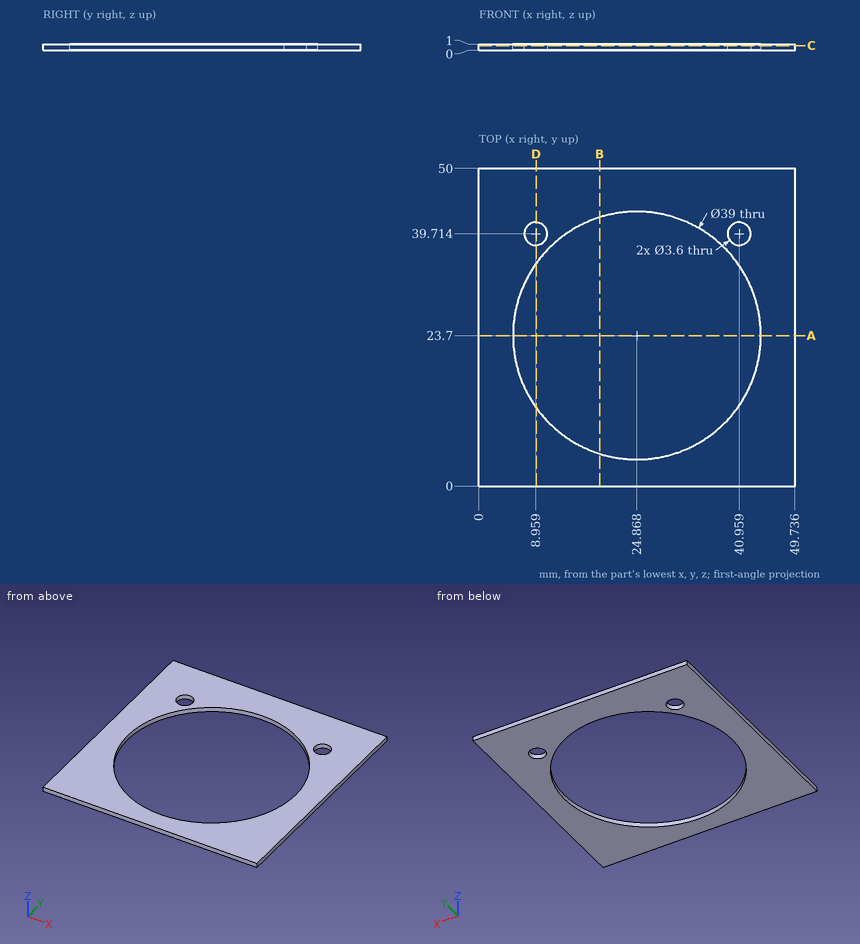
Geometry check sheet. Reference: drawing and pictorial views, mm from the part's lowest x, y, z. Round coordinates to 2 decimals unless told otherwise and drop trailing zeros. Write each loop counter-clockwise with the first axis right and the second up, starting at its lowest first coordinate (ties: lowest second). Pieces come first, ordered by that corner, then holes.
Item 1: Section check B-B (x = 19). Record the boundary of the cut face in (y, z), plus the area to 3 significant figures.
Determined:
outline: (0, 0) - (5.1, 0) - (5.1, 1) - (0, 1) - close; (42.3, 0) - (50, 0) - (50, 1) - (42.3, 1) - close
area: 12.8 mm2
Item 2: Material ranges on line 1 along Y through (x, z) = (8, 0.6) (1 decimal); line 2 along X through (y, z) = (17, 0.6) (1 decimal); line 3 along Y through (x, z) = (34, 0.35), recorded low to high.
Determined:
line 1: y = 0 to 13.9, 33.5 to 38.2, 41.2 to 50
line 2: x = 0 to 6.6, 43.2 to 49.7
line 3: y = 0 to 6.47, 40.93 to 50
Item 3: Section check A-A (y = 23.7). Record the boundary of the cut face in (x, z).
Determined:
outline: (0, 0) - (5.37, 0) - (5.37, 1) - (0, 1) - close; (44.37, 0) - (49.74, 0) - (49.74, 1) - (44.37, 1) - close
Item 4: Section check D-D (x = 9). Record the boundary of the cut face in (y, z) (1 decimal).
Determined:
outline: (0, 0) - (12.4, 0) - (12.4, 1) - (0, 1) - close; (35, 0) - (37.9, 0) - (37.9, 1) - (35, 1) - close; (41.5, 0) - (50, 0) - (50, 1) - (41.5, 1) - close
Item 5: Section check C-C (z = 0.75). Record the boundary of the cut face in (x, y).
Determined:
outline: (0, 0) - (49.74, 0) - (49.74, 50) - (0, 50) - close; hole circle Ø39 at (24.87, 23.7); hole circle Ø3.6 at (8.96, 39.71); hole circle Ø3.6 at (40.96, 39.71)
